Geometry: see drawing. Coordinates: mm, zero at the bounding-box minimum. A direction names the side the tool comes from. Coordinates: 2 decimals unless noted, no trailing zeros. Loops run counter-clockwise (first coordinate to the right, second up) from the corner with the lowest first, then second, coordinate; pieces in that order, holes last. Notation, with made-up numbers: (46, 61.25) -> (57, 61.25) arc R17 cw to (57, 81.25) -> close; hole circle Ø5 at (31, 61). An arc over 180 degrees is marked (long way). One line per question, with ' | ' between items. Start each with the question number.
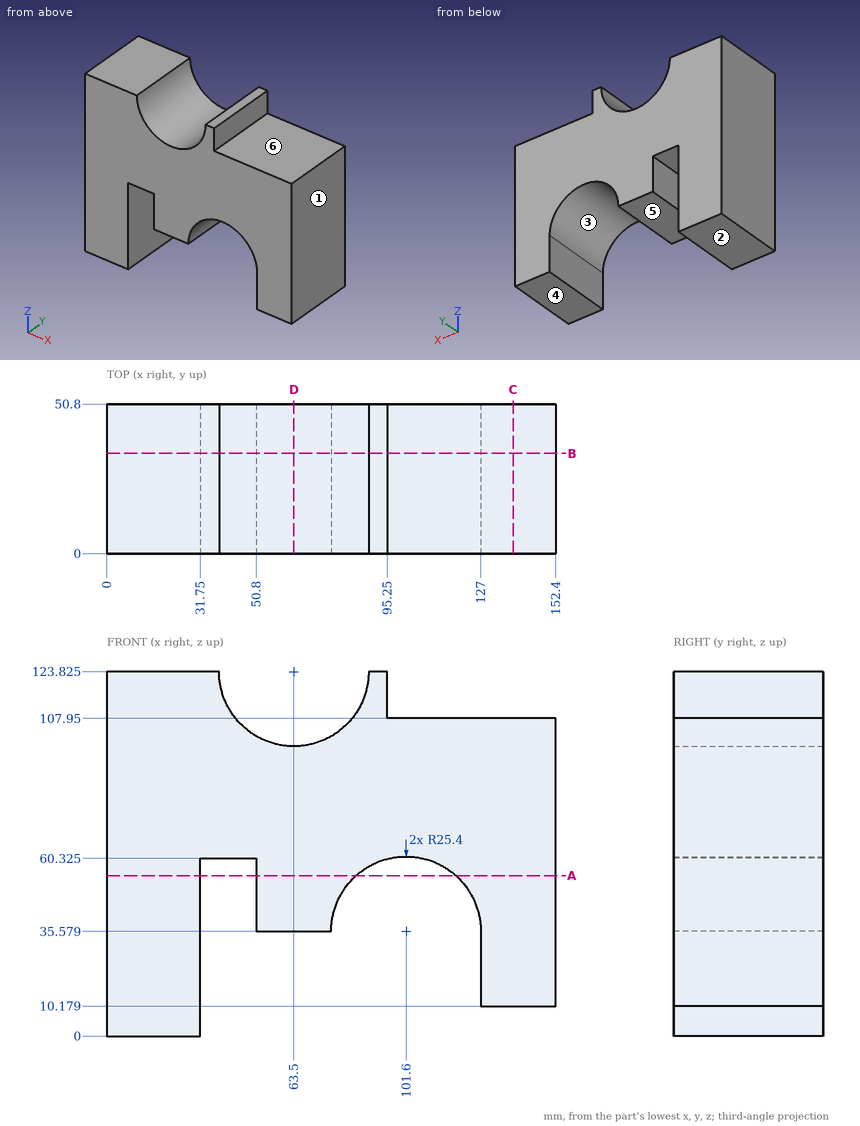
(1) Draft query along X for the marked faces 1, 2 and 3. Return one class per face: pulls with the +X half, pulls with the -X half, needs draft (parallel to the pull), parting line crosses it, or undercut.
(2) Ray query, L1, parallel to X at y = 32, z = 24; L2, parallel to Z at x = 34, y = 16.5 (3 decimals); L3, parallel to X at y = 5.5, z = 47. Return the intervals inside material, ascending.
(3) Contact query for flat-ended pins moving along their axis: pin 1 Ø15 at (x, y) = (42.5, 19.5) entering from -Z (3 decimals); pin 2 Ø8 at (y, z) = (26, 116.5) entering from +X; pin 3 Ø8 at (x, y) = (64.5, 42) entering from +Z. Output: stop coordinate, or through.
(4) Cut plane C-C, the plane x = 138. Return the cut outline in (y, z), and give its area (3 significant figures).
(5) Cut plane A-A, the plane z = 54.5. Return the cut outline in (x, y).
(6) Cut plane B-B, the plane y = 34. Return the cut outline in (x, z) (3 decimals), and give its area (3 significant figures).
(7) Access query for the marked faces 4, 5 and 6. Directions: +Z, -Z, +X, -X, +Y, -Y. A direction counts if a zero-diameter tool reaches every point of the face in a straight line with its end or side. Return the directions, or none.
(8) Cut plane D-D, the plane x = 63.5. Return the cut outline in (y, z) (3 decimals).
Here are the results:
1) face 1: pulls with the +X half | face 2: needs draft | face 3: undercut
2) L1: x = 0 to 31.75, 127 to 152.4 | L2: z = 60.325 to 123.825 | L3: x = 0 to 31.75, 50.8 to 78.91, 124.29 to 152.4
3) pin 1: stops at z = 60.325 | pin 2: stops at x = 95.25 | pin 3: stops at z = 98.92
4) outline: (0, 10.18) -> (50.8, 10.18) -> (50.8, 107.95) -> (0, 107.95) -> close | area: 4,970 mm2
5) outline: (0, 0) -> (31.75, 0) -> (31.75, 50.8) -> (0, 50.8) -> close; (50.8, 0) -> (84.65, 0) -> (84.65, 50.8) -> (50.8, 50.8) -> close; (118.55, 0) -> (152.4, 0) -> (152.4, 50.8) -> (118.55, 50.8) -> close
6) outline: (0, 0) -> (31.75, 0) -> (31.75, 60.325) -> (50.8, 60.325) -> (50.8, 35.579) -> (76.2, 35.579) arc R25.4 cw to (127, 35.579) -> (127, 10.179) -> (152.4, 10.179) -> (152.4, 107.95) -> (95.25, 107.95) -> (95.25, 123.825) -> (88.9, 123.825) arc R25.4 cw to (38.1, 123.825) -> (0, 123.825) -> close | area: 11,800 mm2
7) face 4: -Z, +X, +Y, -Y | face 5: -Z, +Y, -Y | face 6: +Z, +X, +Y, -Y
8) outline: (0, 35.579) -> (50.8, 35.579) -> (50.8, 98.425) -> (0, 98.425) -> close
